Source: CAD feature listing. Evaluate the final solid. Frame: model axes, mm. Face numbers are marked on the shaded views. Coordinates: 2 decimals unless noted, no trailing zeros. Loops run counter-clockwise (first coordinate to the right, second up) from the corner with the lowest first, then second, coordinate; pieces in that order, holes last. Notation, with made-up numbers: (54.25, -3.5) - (98.25, -3.5) arc R21 cw to (98.25, 7.5) - close; hole circle Ø10 at (37, 79.25). An arc over 180 degrees is marked (long way). Use CSV: the item, a comma, the result in double quotes. Start each with the question number.
```python
from build123d import *
from build123d.topology import SkipClean

# Parameters (mm, degrees)
SKETCH2_R           = 25
BOSS_EXTRUDE1_DEPTH = 2.5
SKETCH4_W           = 2.5
SKETCH4_H           = 2.726925283
CUT_EXTRUDE1_DEPTH  = 22.5
SKETCH8_W           = 1
SKETCH8_H           = 1
SKETCH8_W_2         = 2
SKETCH9_W           = 0.5
SKETCH9_H           = 0.5
BOSS_EXTRUDE3_DEPTH = 3.5
SKETCH10_R          = 0.1
CUT_EXTRUDE2_DEPTH  = 17.5
SKETCH11_W          = 2
SKETCH11_H          = 30
BOSS_EXTRUDE4_DEPTH = 15
SKETCH12_R          = 1
SKETCH12_R_2        = 0.25
CUT_EXTRUDE3_DEPTH  = 15


with BuildPart() as part:
    # Sketch2 → Boss-Extrude1 (new body)
    with BuildSketch(Plane(origin=(0, 0, 0), x_dir=(0, 1, 0), z_dir=(0, 0, 1))):
        with Locations(Location((0, 0, 0), (0, 0, 270))):
            Circle(SKETCH2_R)
    extrude(amount=BOSS_EXTRUDE1_DEPTH)

    # Sketch4 → Cut-Extrude1 (cut)
    with BuildSketch(Plane(origin=(0, 0, 0), x_dir=(-1, 0, 0), z_dir=(0, 1, 0))):
        with Locations((1.25, 2.363462641)):
            Rectangle(SKETCH4_W, SKETCH4_H)
    extrude(amount=-CUT_EXTRUDE1_DEPTH, mode=Mode.SUBTRACT)

    # Sketch8 → Revolve2 (revolve)
    with SkipClean():  # the faces are left unmerged after this step: merging them gives an invalid solid
        with BuildSketch(Plane.YZ, mode=Mode.PRIVATE) as revolve2_sk:
            with Locations((2.5, -0.5)):
                Rectangle(SKETCH8_W, SKETCH8_H)
            with Locations((4.5, -0.5)):
                Rectangle(SKETCH8_W, SKETCH8_H)
            with Locations((6.5, -0.5)):
                Rectangle(SKETCH8_W, SKETCH8_H)
            with Locations((8.5, -0.5)):
                Rectangle(SKETCH8_W, SKETCH8_H)
            with Locations((24, -0.5)):
                Rectangle(SKETCH8_W_2, SKETCH8_H)
        revolve(revolve2_sk.sketch.rotate(Axis((0, 0, 0), (0, 0, 1)), 90), axis=Axis((0, 0, 0), (0, 0, 1)))
    add(part.part.scale(1), mode=Mode.REPLACE)  # the faces are merged on a copy

    # Sketch9 → Boss-Extrude3 (add)
    with SkipClean():  # the faces are left unmerged after this step: merging them gives an invalid solid
        with BuildSketch(Plane(origin=(0, 0, 0), x_dir=(0, 1, 0), z_dir=(0, 0, 1))):
            with Locations((-4.75, 1.25)):
                Rectangle(SKETCH9_W, SKETCH9_H)
            with Locations((-9.75, 1.25)):
                Rectangle(SKETCH9_W, SKETCH9_H)
            with Locations((-14.75, 1.25)):
                Rectangle(SKETCH9_W, SKETCH9_H)
            with Locations((-19.75, 1.25)):
                Rectangle(SKETCH9_W, SKETCH9_H)
        extrude(amount=BOSS_EXTRUDE3_DEPTH)

    # Sketch10 → Cut-Extrude2 (cut)
    with SkipClean():  # the faces are left unmerged after this step: merging them gives an invalid solid
        with BuildSketch(Plane.XZ.offset(20)):
            with Locations(Location((-1.25, 3.202014363, 0), (0, 0, 270))):
                Circle(SKETCH10_R)
        extrude(amount=-CUT_EXTRUDE2_DEPTH, mode=Mode.SUBTRACT)

    # Sketch11 → Boss-Extrude4 (add)
    with SkipClean():  # the faces are left unmerged after this step: merging them gives an invalid solid
        with BuildSketch(Plane.XY.offset(2.5)):
            with Locations((18.558520072, 0)):
                Rectangle(SKETCH11_W, SKETCH11_H)
        extrude(amount=BOSS_EXTRUDE4_DEPTH)

    # Sketch12 → Cut-Extrude3 (cut)
    with SkipClean():  # the faces are left unmerged after this step: merging them gives an invalid solid
        with BuildSketch(Plane.YZ.offset(19.558520072)):
            with Locations((12, 10.613168665)):
                Circle(SKETCH12_R)
            with Locations((-12, 10.613168665)):
                Circle(SKETCH12_R)
            with Locations((0.5, 3.229684711)):
                Circle(SKETCH12_R_2)
            with Locations((1.5, 3.229684711)):
                Circle(SKETCH12_R_2)
            with Locations((-1.5, 3.229684711)):
                Circle(SKETCH12_R_2)
            with Locations((-0.5, 3.229684711)):
                Circle(SKETCH12_R_2)
        extrude(amount=-CUT_EXTRUDE3_DEPTH, mode=Mode.SUBTRACT)


solid = part.part
```
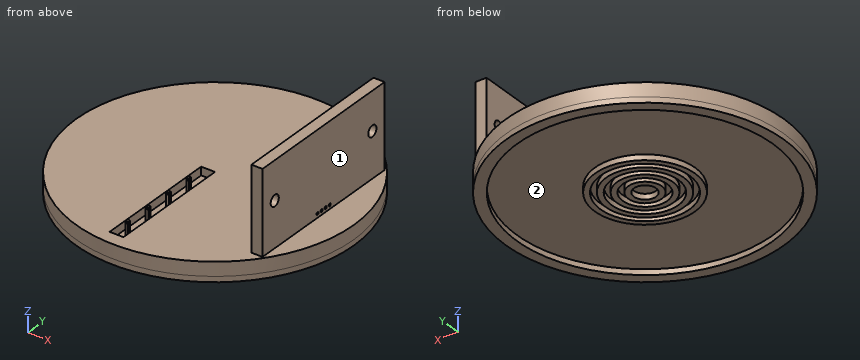
(1) Section A-A on y = 12. Output: boundary loops of the cut face in (x, z).
(2) Draft query along Y for the marked faces 1 and 2. Return one class per face: released by +Y, released by -Y, zero draft, split by the parting line, or undercut.
(3) Section C-C on x = 20.5. Output: boundary loops of the cut face in (y, z).
(4) Section B-B on x = -14.5. Output: boundary loops of the cut face in (y, z).
(5) Ray query, line 1 (Z direction, x = -20.5, y = 3.5); line 2 (Z direction, x = 18, y = 15.5); line 3 (X direction, y = -9, z = 16.25). Return the intervals inside material, ascending. Write a range as [from, to].
(6) Pin query (flat end, axial travel): pin 1 Ø4.5 at (y, z) = (-6.5, 9.5) entering from -X; pin 2 Ø0.8 at (y, z) = (-17, 2) entering from -X; pin 3 Ø6 at (y, z) = (-19.5, 2) entering from -X; pin 4 Ø4 at (y, z) = (17.5, 5) entering from -X. Return the tip coordinate at first contact, or that it passes through.
Solution:
1,outline,"(-21.93, -1) - (-19.62, -1) - (-19.62, 0) - (19.62, 0) - (19.62, -1) - (21.93, -1) - (21.93, 2.5) - (19.56, 2.5) - (19.56, 9.61) - (17.56, 9.61) - (17.56, 2.5) - (-21.93, 2.5) - close; (17.56, 11.61) - (19.56, 11.61) - (19.56, 17.5) - (17.56, 17.5) - close"
2,face 1,"zero draft"
2,face 2,"undercut"
3,outline,"(-14.31, -1) - (-10.43, -1) - (-10.43, 0) - (10.43, 0) - (10.43, -1) - (14.31, -1) - (14.31, 2.5) - (-14.31, 2.5) - close"
4,outline,"(-20.37, -1) - (-17.85, -1) - (-17.85, 0) - (17.85, 0) - (17.85, -1) - (20.37, -1) - (20.37, 2.5) - (-20.37, 2.5) - close"
5,line 1,"z = [0, 2.5]"
5,line 2,"z = [-1, 2.5]"
5,line 3,"x = [17.56, 19.56]"
6,pin 1,"stops at x = 17.56"
6,pin 2,"stops at x = -18.69"
6,pin 3,"stops at x = -18.78"
6,pin 4,"passes through"
